Check sheet for the modelled part. Datum: model origin and axes. Units: mm. Give positions to 0.01 mm unless a question says otherwise; leave off trailing zeros. Order: outer loops, then holes, each group sorted by start corner. A loop starts at its lowest first (then second) coordinate and runs counter-clockwise, first axis right, second up.
from build123d import *

# Parameters (mm, degrees)
SKETCH_1_R          = 10
EXTRUDE_1_DEPTH     = 1000
SKETCH_2_R          = 2.75
CUT_EXTRUDE_2_DEPTH = 450


with BuildPart() as part:
    # 草图1 → 凸台-拉伸1 (new body)
    with BuildSketch(Plane.XY):
        with Locations((0, 27)):
            Circle(SKETCH_1_R)
        with BuildLine():
            Line((-22.5, 5), (-22.5, 0))
            Line((-22.5, 0), (0, 0))
            Line((0, 0), (0, 17))
            ThreePointArc((0, 17), (-1.870828693, 17.176558648), (-3.67559519, 17.7))
            Line((-3.67559519, 17.7), (-4, 17.7))
            Line((-4, 17.7), (-9.5, 10))
            Line((-9.5, 10), (-9.5, 5))
            Line((-9.5, 5), (-22.5, 5))
        make_face()
        with BuildLine():
            Line((0, 17), (0, 0))
            Line((0, 0), (22.5, 0))
            Line((22.5, 0), (22.5, 5))
            Line((22.5, 5), (9.5, 5))
            Line((9.5, 5), (9.5, 10))
            Line((9.5, 10), (4, 17.7))
            Line((4, 17.7), (3.67559519, 17.7))
            ThreePointArc((3.67559519, 17.7), (1.870828693, 17.176558648), (0, 17))
        make_face()
    extrude(amount=EXTRUDE_1_DEPTH)

    # 草图2 → 切除-拉伸2 (cut)
    with BuildSketch(Plane(origin=(0, 0, 0), x_dir=(1, 0, 0), z_dir=(0, 1, 0))):
        with Locations((15, -500)):
            Circle(SKETCH_2_R)
        with Locations((15, -650)):
            Circle(SKETCH_2_R)
        with Locations(Location((-15, -500, 0), (0, 0, 180))):
            Circle(SKETCH_2_R)
        with Locations(Location((-15, -650, 0), (0, 0, 180))):
            Circle(SKETCH_2_R)
        with Locations((15, -350)):
            Circle(SKETCH_2_R)
        with Locations(Location((-15, -350, 0), (0, 0, 180))):
            Circle(SKETCH_2_R)
        with Locations(Location((-15, -200, 0), (0, 0, 180))):
            Circle(SKETCH_2_R)
        with Locations((15, -200)):
            Circle(SKETCH_2_R)
        with Locations(Location((-15, -50, 0), (0, 0, 180))):
            Circle(SKETCH_2_R)
        with Locations((15, -50)):
            Circle(SKETCH_2_R)
        with Locations(Location((-15, -800, 0), (0, 0, 180))):
            Circle(SKETCH_2_R)
        with Locations((15, -800)):
            Circle(SKETCH_2_R)
        with Locations(Location((-15, -950, 0), (0, 0, 180))):
            Circle(SKETCH_2_R)
        with Locations((15, -950)):
            Circle(SKETCH_2_R)
    extrude(amount=CUT_EXTRUDE_2_DEPTH, mode=Mode.SUBTRACT)


solid = part.part
1) Depth check by flat-ended pin: pin 1 Ø10 at (x, z) = (8, 552.5) entering from +Y; pin 2 Ø6 at (x, z) = (5, 412.5) entering from +Y; pin 3 Ø1 at (x, z) = (9, 519.5) entering from +Y. Enter the tip coordinate at first touch or a pass-through.
Recorded:
pin 1: stops at y = 36.54
pin 2: stops at y = 36.8
pin 3: stops at y = 32.27
2) Draft check along Y on faces 1 (the face through (0, 37, 493)), 2 (the face through (0, 15, 0)), 3 (the face through (0, 0, 493)). Enter one of: +Y half, -Y half, draft (parallel to the pull), parting line (faces both ways), or undercut.
Recorded:
face 1: undercut
face 2: draft
face 3: -Y half
3) Material ranges on L1, parallel to X at y = 1, z = 650; L2, parallel to Y at x = -14, z = 695; L3, parallel to X at y = 5.5, z = 656.5, recorded low to high.
Recorded:
L1: x = -22.5 to -17.75, -12.25 to 12.25, 17.75 to 22.5
L2: y = 0 to 5
L3: x = -9.5 to 9.5
4) Section check A-A, the plane y = 27. Record the cut outline in (x, z), then the cut area to 3 significant figures.
Recorded:
outline: (-10, 0) - (10, 0) - (10, 1000) - (-10, 1000) - close
area: 20,000 mm2
